Autodesk Inventor part; units mm, degrees
ref_plane "YZ Plane" through (0, 0, 0) normal (1, 0, 0) x (0, 1, 0)
ref_plane "XZ Plane" through (0, 0, 0) normal (0, 1, 0) x (-1, 0, 0)
ref_plane "XY Plane" through (0, 0, 0) normal (0, 0, 1) x (1, 0, 0)
sketch "Skizze1" plane through (0, 0, 0) normal (0, 1, 0) x (-1, 0, 0)
  circle A0 centre (0, 0) radius 25.4
  dimension "d0" = 50.8
extrude "Extrusion1" add sketch "Skizze1" along normal blind 2
sketch "Skizze2" plane through (0, 0, 0) normal (0, -1, 0) x (1, 0, 0)
  circle A0 centre (0, 0) radius 25.4
  line L0 (-20.6475, 0) -> (0, 20.6475) construction
  line L1 (0, 20.6475) -> (20.6475, 0) construction
  line L2 (20.6475, 0) -> (0, -20.6475) construction
  line L3 (0, -20.6475) -> (-20.6475, 0) construction
  line L4 (0, 0) -> (10.3238, 10.3238) construction
  line L5 (0, 0) -> (-10.3238, 10.3238) construction
  circle A1 centre (0, 0) radius 25.4 construction
  line L6 (0, 0) -> (0, 25.4) construction
  point P0 (-20.6475, 0)
  point P1 (0, 20.6475)
  point P2 (20.6475, 0)
  dimension "d3" = 29.2
  dimension "d4" = 29.2
  dimension "d63" = 45
hole "Bohrung1" at (-20.6475, 0, 0) at (0, 0, 20.6475) at (20.6475, 0, 0) at (0, 0, -20.6475) direction (0, 1, 0) diameter 3 end through all countersink diameter 6 countersink angle 90
sketch "Skizze9" plane through (0, 0, 0) normal (0, -1, 0) x (1, 0, 0)
  circle A0 centre (0, 0) radius 25.4
  circle A1 centre (0, 0) radius 11
  dimension "d53" = 22
extrude "Extrusion7" cut sketch "Skizze9" against normal up to next contours A1
sketch "Skizze7" plane through (0, 0, 0) normal (0, -1, 0) x (1, 0, 0)
  circle A0 centre (0, 0) radius 25.4 construction
  line L0 (-9.9, 9.9) -> (9.9, 9.9) construction
  line L1 (9.9, 9.9) -> (9.9, -9.9) construction
  line L2 (9.9, -9.9) -> (-9.9, -9.9) construction
  line L3 (-9.9, -9.9) -> (-9.9, 9.9) construction
  line L4 (-9.9, 0) -> (9.9, 0) construction
  dimension "d42" = 19.8
  dimension "d43" = 19.8
hole "Bohrung3" at (-9.9, 0, 9.9) at (9.9, 0, -9.9) direction (0, 1, 0) diameter 3 end through all countersink diameter 6 countersink angle 90
sketch "Skizze10" plane through (0, 0, 0) normal (0, -1, 0) x (1, 0, 0)
  circle A0 centre (0, 0) radius 25.4
  line L0 (-12.55, 16.2) -> (12.55, 16.2)
  line L1 (12.55, 16.2) -> (12.55, -12.5)
  line L2 (12.55, -12.5) -> (-12.55, -12.5)
  line L3 (-12.55, -12.5) -> (-12.55, 16.2)
  line L4 (0, 16.2) -> (0, -12.5) construction
  line L5 (-7, -12.5) -> (-5, -12.5) construction
  line L6 (-5, -12.5) -> (-5, -14.5)
  line L7 (-5, -14.5) -> (-7, -14.5)
  line L8 (-7, -14.5) -> (-7, -12.5)
  line L9 (5, -12.5) -> (7, -12.5) construction
  line L10 (7, -12.5) -> (7, -14.5)
  line L11 (7, -14.5) -> (5, -14.5)
  line L12 (5, -14.5) -> (5, -12.5)
  line L13 (-5, -12.5) -> (5, -12.5) construction
  dimension "d56" = 25.1
  dimension "d57" = 28.7
  dimension "d58" = 12.5
  dimension "d59" = 2
  dimension "d60" = 2
  dimension "d61" = 10
  dimension "d62" = 2
properties part number "anschluss_daten"
Design review of the part built by this model. Coordinates are the model's own, in mm. Coordinates: 2 decimals unless noted, no trailing zeros. Loops run counter-clockwise (first coordinate to the right, second up) from the corner with the lowest first, then second, coordinate; pieces in that order, holes last.
Q1. We need section D-D on z = 9.9. State the section outline as (x, y) points, and give its area (3 significant figures).
Reported:
outline: (-23.39, 0) - (-12.9, 0) - (-11.4, 1.5) - (-11.4, 2) - (-23.39, 2) - close; (-8.4, 1.5) - (-6.9, 0) - (-4.79, 0) - (-4.79, 2) - (-8.4, 2) - close; (4.79, 0) - (23.39, 0) - (23.39, 2) - (4.79, 2) - close
area: 66.1 mm2
Q2. We need section A-A on z = 0. State the section outline as (x, y) points.
Reported:
outline: (-25.4, 0) - (-23.65, 0) - (-22.15, 1.5) - (-22.15, 2) - (-25.4, 2) - close; (-19.15, 1.5) - (-17.65, 0) - (-11, 0) - (-11, 2) - (-19.15, 2) - close; (11, 0) - (17.65, 0) - (19.15, 1.5) - (19.15, 2) - (11, 2) - close; (22.15, 1.5) - (23.65, 0) - (25.4, 0) - (25.4, 2) - (22.15, 2) - close
Q3. The part is to be moulded in two halves that separate along Z. For faces 1 (the face through (-11, 0, -5)), 2 (the face through (5.506, 0.986, 24.796)), 3 (the face through (22.11, 1.75, 0.33)), 4 (the face through (-11.165, 1.754, 9.094)), say which applies: +Z half, -Z half, draft (parallel to the pull), parting line (faces both ways), or undercut.
Reported:
face 1: draft
face 2: parting line
face 3: undercut
face 4: undercut
Q4. To check wall thickness, follow line 1 (Z direction, x = 0, y = 1.7); line 2 (X direction, y = 1.75, z = 9.9); line 3 (Z direction, x = 0, y = 0.15). State the ranges of each line that lie inside material, in increasing order.
Reported:
line 1: z = -25.4 to -22.15, -19.15 to -11, 11 to 19.15, 22.15 to 25.4
line 2: x = -23.39 to -11.4, -8.4 to -4.79, 4.79 to 23.39
line 3: z = -25.4 to -23.5, -17.8 to -11, 11 to 17.8, 23.5 to 25.4
Q5. We need section B-B on x = 9.9. State the section outline as (y, z) points.
Reported:
outline: (0, -23.39) - (2, -23.39) - (2, -11.4) - (1.5, -11.4) - (0, -12.9) - close; (0, -6.9) - (1.5, -8.4) - (2, -8.4) - (2, -4.79) - (0, -4.79) - close; (0, 4.79) - (2, 4.79) - (2, 23.39) - (0, 23.39) - close
Q6. We need section C-C on y = 0.6. State the section outline as (x, z) points.
Reported:
outline: circle Ø50.8 at (0, 0); hole circle Ø4.8 at (-20.65, 0); hole circle Ø4.8 at (-9.9, 9.9); hole circle Ø22 at (0, 0); hole circle Ø4.8 at (0, -20.65); hole circle Ø4.8 at (0, 20.65); hole circle Ø4.8 at (9.9, -9.9); hole circle Ø4.8 at (20.65, 0)
Q7. For pin 1 (1.5 mm diameter, centred on x = -8.5, z = 2.5, fed in from +Y); pin 2 (5 mm diameter, centred on x = 9.9, z = -9.9, fed in from -Y), all flat-tipped, find the tip position at first contact; note any pin that passes through.
Reported:
pin 1: passes through
pin 2: stops at y = 0.5
